The model under review builds one solid part; all positions refer to its coordinate system, in mm. Face numbers are marked on the shaded views. A direction names the side the tool comes from. Coordinates: 2 decimals unless noted, no trailing zeros. Write each loop counter-clockwise with the first axis right and the second up, starting at its lowest first coordinate (ties: lowest second). Pieces come first, ordered by that corner, then holes. Notation, with made-up numbers: (78, 83.5) - (118, 83.5) arc R29 cw to (118, 108.5) - close; hole circle Ø5 at (69.25, -35.5). An arc over 180 degrees is marked (long way). Put each result on its own line as item: value.
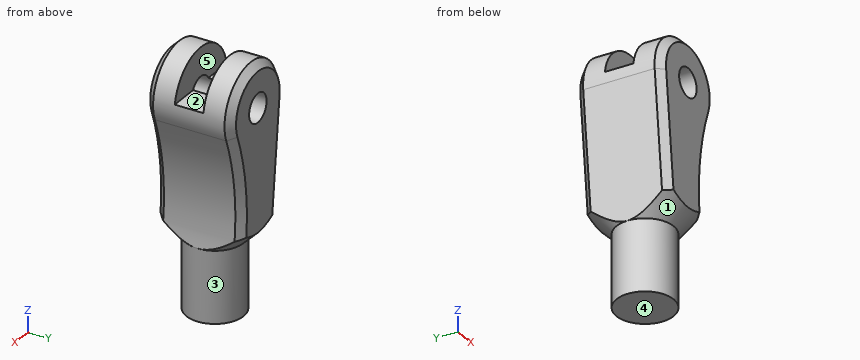
from build123d import *

# Parameters (mm, degrees)
SKETCH_R        = 10
PAD_DEPTH       = 40
SKETCH001_W     = 20
SKETCH001_H     = 4
POCKET_DEPTH    = 10
SKETCH003_R     = 10
SKETCH003_R_2   = 4
POCKET001_DEPTH = 10
SKETCH005_R     = 2
POCKET002_DEPTH = 38.001
SKETCH006_W     = 45.010599
SKETCH006_H     = 48.069569
POCKET003_DEPTH = 4.001
SKETCH009_W     = 22.304068
SKETCH009_H     = 42.809419
POCKET004_DEPTH = 4.001
CHAMFER_SIZE    = 1
CHAMFER001_SIZE = 1


with BuildPart() as part:
    # Sketch → Pad (new body)
    with BuildSketch(Plane.XY):
        Circle(SKETCH_R)
    extrude(amount=PAD_DEPTH)

    # Sketch001 (on Face3 of Pad) → Pocket (cut)
    with BuildSketch(Plane.XY.offset(40)):
        Rectangle(SKETCH001_W, SKETCH001_H)
    extrude(amount=-POCKET_DEPTH, mode=Mode.SUBTRACT)

    # Sketch003 (on Face2 of Pocket) → Pocket001 (cut)
    with BuildSketch(Plane(origin=(0, 0, 0), x_dir=(1, 0, 0), z_dir=(0, 0, -1))):
        Circle(SKETCH003_R)
        Circle(SKETCH003_R_2, mode=Mode.SUBTRACT)
    extrude(amount=-POCKET001_DEPTH, mode=Mode.SUBTRACT)

    # Sketch005 (on DatumPlane) → Pocket002 (cut, through all)
    with BuildSketch(Plane.XZ.offset(28)):
        with Locations((0, 29.052325)):
            Circle(SKETCH005_R)
        with BuildLine():
            ThreePointArc((5.607622, 26.918181), (0.769749, 35.002744), (-5.966094, 28.415363))
            Line((-5.966094, 28.415363), (-4, 10))
            Line((-4, 10), (-20.111568, 10))
            Line((-20.111568, 10), (-20.111568, 42.267994))
            Line((-20.111568, 42.267994), (18.230141, 42.267994))
            Line((18.230141, 42.267994), (18.230141, 10))
            Line((18.230141, 10), (4, 10))
            ThreePointArc((5.607622, 26.918181), (3.659522, 18.567825), (4, 10))
        make_face()
    extrude(amount=-POCKET002_DEPTH, mode=Mode.SUBTRACT)

    # Sketch006 (on DatumPlane) → Pocket003 (cut, through all)
    with BuildSketch(Plane(origin=(0, -6, 0), x_dir=(-1, 0, 0), z_dir=(0, 1, 0))):
        with Locations((-1.18355, 18.119115)):
            Rectangle(SKETCH006_W, SKETCH006_H)
    extrude(amount=-POCKET003_DEPTH, mode=Mode.SUBTRACT)

    # Sketch008 → Groove (revolve, cut)
    with BuildSketch(Plane.XZ):
        Polygon((-4, 10), (-11.309977, 17.309977), (-11.309977, 10), align=None)
    revolve(axis=Axis((0, 0, 0), (0, 0, 1)), mode=Mode.SUBTRACT)

    # Sketch009 (on DatumPlane) → Pocket004 (cut, through all)
    with BuildSketch(Plane.XZ.offset(-6)):
        with Locations((-2.652106, 20.426258)):
            Rectangle(SKETCH009_W, SKETCH009_H)
    extrude(amount=-POCKET004_DEPTH, mode=Mode.SUBTRACT)

    # Chamfer
    chamfer_edges = [part.edges().sort_by_distance(p)[0] for p in [
        (3.83859, -6, 20.072708),
        (0.769749, -6, 35.002744),
        (-5.165605, -6, 20.917609),
    ]]
    chamfer(chamfer_edges, length=CHAMFER_SIZE)

    # Chamfer001
    chamfer001_edges = [part.edges().sort_by_distance(p)[0] for p in [
        (3.83859, 6, 20.072708),
        (0.769749, 6, 35.002744),
        (-5.165605, 6, 20.917609),
    ]]
    chamfer(chamfer001_edges, length=CHAMFER001_SIZE)


solid = part.part
1. Machinability: for the marked faces 1 and 2, which of the approach directions +Z, -Z, +X, -X, +Y, -Y give a long, thin tool a straight path to every point of the face, cutting with its end or side? Answer none if there is none.
Determined:
face 1: -Z, -Y
face 2: +Z, +X, -X
2. For pin 1 Ø6 at (y, z) = (1, 21) entering from +X; pin 2 Ø1 at (x, y) = (-1, 3.5) entering from -Z; pin 3 Ø1.5 at (x, y) = (-4, -1) entering from +Z; pin 4 Ø3 at (y, z) = (4, 24.5) entering from -X, all flat-tipped, find the tip position at first contact; note any pin that passes through.
Determined:
pin 1: stops at x = 4.65
pin 2: stops at z = 0
pin 3: stops at z = 30
pin 4: stops at x = -5.71
3. Consider section A-A on x = 0. State the section outline as (y, z) points, plus the area to 3 significant figures.
Determined:
outline: (-6, 12) - (-4, 10) - (-4, 0) - (4, 0) - (4, 10) - (6, 12) - (6, 27.05) - (-6, 27.05) - close; (-6, 31.05) - (-2, 31.05) - (-2, 35.05) - (-5, 35.05) - (-6, 34.05) - close; (2, 31.05) - (6, 31.05) - (6, 34.05) - (5, 35.05) - (2, 35.05) - close
area: 312 mm^2
4. To check wall thickness, follow probe 1 along Z at (x, y) = (0, 2.25); probe 2 along Z at (x, y) = (0, -1); probe 3 along X at (y, z) = (0.25, 4). State the ranges of each line that lie inside material, in increasing order.
Determined:
probe 1: z = 0 to 27.05, 31.05 to 35.05
probe 2: z = 0 to 27.05
probe 3: x = -3.99 to 3.99
5. The part is to be moulded in two halves that separate along Y. For the marked faces 3, 4 and 5, say which applies: +Y half, -Y half, draft (parallel to the pull), parting line (faces both ways), or undercut.
Determined:
face 3: parting line
face 4: draft
face 5: undercut
